```python
from build123d import *

# Parameters (mm, degrees)
SALIENTE_EXTRUIR1_DEPTH = 600


with BuildPart() as part:
    # Croquis1 → Saliente-Extruir1 (new body)
    with BuildSketch(Plane(origin=(0, 0, 0), x_dir=(1, 0, 0), z_dir=(0, 1, 0))):
        with BuildLine():
            Line((0, 2.5), (0, 0))
            Line((0, 0), (10.5, 0))
            Line((10.5, 0), (10.5, 20))
            Line((10.5, 20), (0, 20))
            Line((0, 20), (0, 17.5))
            ThreePointArc((0, 17.5), (-0.146446609, 17.146446609), (-0.5, 17))
            Line((-0.5, 17), (-1, 17))
            ThreePointArc((-1, 17), (-1.828095708, 10), (-1, 3))
            Line((-1, 3), (-0.5, 3))
            ThreePointArc((-0.5, 3), (-0.146446609, 2.853553391), (0, 2.5))
        make_face()
        with BuildLine():
            Line((10.5, 20), (10.5, 0))
            Line((10.5, 0), (21, 0))
            Line((21, 0), (21, 2.5))
            ThreePointArc((21, 2.5), (21.146446609, 2.853553391), (21.5, 3))
            Line((21.5, 3), (22, 3))
            Line((22, 3), (22, 17))
            Line((22, 17), (21.5, 17))
            ThreePointArc((21.5, 17), (21.146446609, 17.146446609), (21, 17.5))
            Line((21, 17.5), (21, 20))
            Line((21, 20), (10.5, 20))
        make_face()
    extrude(amount=SALIENTE_EXTRUIR1_DEPTH)


solid = part.part
```
Geometry: final body of the model. Coordinates: model frame, mm. Coordinates: 2 decimals unless noted, no trailing zeros. Loops run counter-clockwise (first coordinate to the right, second up) from the corner with the lowest first, then second, coordinate; pieces in that order, holes last. Notation, with made-up numbers: (16.25, 33) -> (35.25, 33) arc R20 cw to (35.25, 55) -> close; hole circle Ø6 at (27.25, -4). An arc over 180 degrees is marked (long way). Use a Markdown table: item, result. Add a question column.
(1) Pin query (flat end, axial travel): pin 1 Ø6 at (y, z) = (132, -17) entering from -X; pin 2 Ø2 at (y, z) = (208, -3) entering from -X; pin 3 Ø0.6 at (x, y) = (21.5, 398.5) entering from -Z. Return the tip coordinate at first contact, or that it passes through.
(2) Line query: line 1 along X through (y, z) = (225, -8); line 2 along Z through (x, y) = (-0.25, 383.5); line 3 along X through (y, z) = (337.5, -2.75). Output: solid intervals per line, ascending.
(3) Section query A-A, the plane y = 463.5. Return loops of the section in (x, z), plus the area to 3 significant figures.
Answer:
| question | item | result |
|---|---|---|
| 1 | pin 1 | stops at x = -1.56 |
| 1 | pin 2 | stops at x = -1.22 |
| 1 | pin 3 | stops at z = -17.1 |
| 2 | line 1 | x = -1.76 to 22 |
| 2 | line 2 | z = -17.07 to -2.93 |
| 2 | line 3 | x = -0.07 to 21.07 |
| 3 | outline | (-1, -17) -> (-0.5, -17) arc R0.5 cw to (0, -17.5) -> (0, -20) -> (21, -20) -> (21, -17.5) arc R0.5 cw to (21.5, -17) -> (22, -17) -> (22, -3) -> (21.5, -3) arc R0.5 cw to (21, -2.5) -> (21, 0) -> (0, 0) -> (0, -2.5) arc R0.5 cw to (-0.5, -3) -> (-1, -3) arc R30 ccw to start |
| 3 | area | 456 mm^2 |
